Input: part model. Units: mm. Frame: model coordinates. A direction names the side the tool comes from. Coordinates: 2 decimals unless noted, no trailing zeros. Order: outer loops, then holes, each group sorted by start corner. A loop starts at its lowest first (then second) coordinate and runs counter-clockwise, first axis right, second up. Notation, with made-up numbers: M 23,53 L 56,53 A22 ccw 56,76 Z; hole C 1.5,69.25 d10. An arc over 180 degrees is marked long. Answer in a Markdown table with one row per item.
from build123d import *

# Parameters (mm, degrees)
SKETCH_1_W          = 174
SKETCH_1_H          = 80
EXTRUDE_1_DEPTH     = 4
SKETCH_3_W          = 4
SKETCH_3_H          = 20
CUT_EXTRUDE_1_DEPTH = 4
SKETCH_4_W          = 50
SKETCH_4_H          = 4
CUT_EXTRUDE_2_DEPTH = 4
SKETCH_5_W          = 2
SKETCH_5_H          = 80
CUT_EXTRUDE_3_DEPTH = 10
SKETCH_6_W          = 50
SKETCH_6_H          = 4
CUT_EXTRUDE_4_DEPTH = 4


with BuildPart() as part:
    # 스케치1 → 보스-돌출1 (new body)
    with BuildSketch(Plane(origin=(0, 0, 0), x_dir=(0, 0, -1), z_dir=(1, 0, 0))):
        Rectangle(SKETCH_1_W, SKETCH_1_H)
    extrude(amount=EXTRUDE_1_DEPTH)

    # 스케치3 → 컷-돌출1 (cut)
    with BuildSketch(Plane(origin=(4, 0, 0), x_dir=(0, 0, -1), z_dir=(1, 0, 0))):
        with Locations((85, 30)):
            Rectangle(SKETCH_3_W, SKETCH_3_H)
        with Locations((85, -30)):
            Rectangle(SKETCH_3_W, SKETCH_3_H)
    extrude(amount=-CUT_EXTRUDE_1_DEPTH, mode=Mode.SUBTRACT)

    # 스케치4 → 컷-돌출2 (cut)
    with BuildSketch(Plane(origin=(4, 0, 0), x_dir=(0, 0, -1), z_dir=(1, 0, 0))):
        with Locations((-2, 38)):
            Rectangle(SKETCH_4_W, SKETCH_4_H)
    extrude(amount=-CUT_EXTRUDE_2_DEPTH, mode=Mode.SUBTRACT)

    # 스케치5 → 컷-돌출3 (cut)
    with BuildSketch(Plane(origin=(4, 0, 0), x_dir=(0, 0, -1), z_dir=(1, 0, 0))):
        with Locations((-86, 0)):
            Rectangle(SKETCH_5_W, SKETCH_5_H)
    extrude(amount=-CUT_EXTRUDE_3_DEPTH, mode=Mode.SUBTRACT)

    # 스케치6 → 컷-돌출4 (cut)
    with BuildSketch(Plane(origin=(4, 0, 0), x_dir=(0, 0, -1), z_dir=(1, 0, 0))):
        with Locations((-3, -6)):
            Rectangle(SKETCH_6_W, SKETCH_6_H)
    extrude(amount=-CUT_EXTRUDE_4_DEPTH, mode=Mode.SUBTRACT)


solid = part.part
1) Mould query, pull axis Z, two halves, no side actions, for faces 1 (the face through (2, 0, -87)), 2 (the face through (2, 38, 27)), 3 (the face through (2, -1, 85)), 4 (the face through (2, -20, -85)). Classes: +Z half, -Z half, draft (parallel to the pull), parting line (faces both ways), or undercut.
Resolved:
| item | result |
|---|---|
| face 1 | -Z half |
| face 2 | undercut |
| face 3 | +Z half |
| face 4 | draft |
2) Cut plane B-B, the plane x = 1.3. Output: boundary loops of the cut face in (y, z).
Resolved:
| item | result |
|---|---|
| outline | M -40,-83 L -20,-83 L -20,-87 L 20,-87 L 20,-83 L 40,-83 L 40,-23 L 36,-23 L 36,27 L 40,27 L 40,85 L -40,85 Z; hole M -8,-22 L -4,-22 L -4,28 L -8,28 Z |
3) Material intervals for probe 1 along Y at (x, z) = (0.2, -18); probe 2 along Z at (x, y) = (0.2, -28), sorted ascending.
Resolved:
| item | result |
|---|---|
| probe 1 | y = -40 to -8, -4 to 36 |
| probe 2 | z = -83 to 85 |
4) Cut plane C-C, the plane y = -34.5. Output: boundary loops of the cut face in (x, z), and give its area (3 significant figures).
Resolved:
| item | result |
|---|---|
| outline | M 0,-83 L 4,-83 L 4,85 L 0,85 Z |
| area | 672 mm2 |
5) Cut plane A-A, the plane z = -2. Output: boundary loops of the cut face in (x, y), and give its area (3 significant figures).
Resolved:
| item | result |
|---|---|
| outline | M 0,-40 L 4,-40 L 4,-8 L 0,-8 Z; M 0,-4 L 4,-4 L 4,36 L 0,36 Z |
| area | 288 mm2 |
6) Reachability of faces 5 (the face through (2, -6, 28)), 6 (the face through (2, 30, -83)), 7 (the face through (2, 38, -23)), 8 (the face through (2, -30, -83)) from +Z, -Z, +X, -X, +Y, -Y: full face, straight path, thin tool, end or side. Return the list, or none.
Resolved:
| item | result |
|---|---|
| face 5 | +X, -X |
| face 6 | -Z, +X, -X, +Y |
| face 7 | +X, -X, +Y |
| face 8 | -Z, +X, -X, -Y |
7) Contact query for flat-ended pins moving along their axis: pin 1 (2 mm diameter, centred on x = 1, y = 38.5, fed in from -Z); pin 2 (2 mm diameter, centred on x = 1.5, z = 13, fed in from +Y). Output: stop coordinate, or through.
Resolved:
| item | result |
|---|---|
| pin 1 | stops at z = -83 |
| pin 2 | stops at y = 36 |
